The model under review builds one solid part; all positions refer to its coordinate system, in mm. A direction names the side the tool comes from. Coordinates: 2 decimals unless noted, no trailing zeros. Order: outer loops, then holes, each group sorted by start corner. A loop starts at its lowest first (then second) coordinate and runs counter-clockwise, first axis right, second up. Notation, with made-up numbers: M 42.25,-10.5 L 55.25,-10.5 A19 ccw 55.25,11.5 Z; hole C -28,0 d3. An arc over 180 degrees is marked long. Answer in a Markdown table with one row per item.
from build123d import *

# Parameters (mm, degrees)
BOSS_EXTRUDE1_DEPTH = 20
SKETCH1_3_W         = 5.45
SKETCH1_3_H         = 16
SKETCH1_3_R         = 1
SKETCH1_3_W_2       = 4
SKETCH1_3_H_2       = 10
BOSS_EXTRUDE2_DEPTH = 2


with BuildPart() as part:
    # Sketch1 → Boss-Extrude1 (new body)
    # profile 1 of 2: a face of its own
    with BuildSketch(Plane(origin=(0, 0, 0), x_dir=(1, 0, 0), z_dir=(0, 1, 0))):
        with BuildLine():
            Line((-0.906603032, 3.2), (-0.906603032, 2.43874968))
            ThreePointArc((-0.906603032, 2.43874968), (1.204646468, 1.952562419), (2.143396968, 0))
            Line((2.143396968, 0), (6.193396968, 0))
            Line((6.193396968, 0), (6.193396968, 8))
            Line((6.193396968, 8), (6.193396968, 13.2))
            Line((6.193396968, 13.2), (-0.906603032, 13.2))
            Line((-0.906603032, 13.2), (-0.906603032, 3.2))
        make_face()
        with BuildLine():
            Line((5.393396968, 12.4), (5.393396968, 0.4))
            Line((5.393396968, 0.4), (2.919064839, 0.4))
            ThreePointArc((2.919064839, 0.4), (1.922948491, 2.386135967), (-0.106603032, 3.290516677))
            Line((-0.106603032, 3.290516677), (-0.106603032, 12.4))
            Line((-0.106603032, 12.4), (5.393396968, 12.4))
        make_face(mode=Mode.SUBTRACT)
    # profile 2 of 2: a face of its own
    with BuildSketch(Plane(origin=(0, 0, 0), x_dir=(1, 0, 0), z_dir=(0, 1, 0))):
        with BuildLine():
            Line((6.193396968, 0), (2.143396968, 0))
            ThreePointArc((2.143396968, 0), (1.204646468, -1.952562419), (-0.906603032, -2.43874968))
            Line((-0.906603032, -2.43874968), (-0.906603032, -3.2))
            Line((-0.906603032, -3.2), (-0.906603032, -13.2))
            Line((-0.906603032, -13.2), (6.193396968, -13.2))
            Line((6.193396968, -13.2), (6.193396968, -8))
            Line((6.193396968, -8), (6.193396968, 0))
        make_face()
        with BuildLine():
            Line((5.393396968, -12.4), (-0.106603032, -12.4))
            Line((-0.106603032, -12.4), (-0.106603032, -3.290516677))
            ThreePointArc((-0.106603032, -3.290516677), (1.922948491, -2.386135967), (2.919064839, -0.4))
            Line((2.919064839, -0.4), (5.393396968, -0.4))
            Line((5.393396968, -0.4), (5.393396968, -12.4))
        make_face(mode=Mode.SUBTRACT)
    extrude(amount=BOSS_EXTRUDE1_DEPTH)

    # Sketch1_3 → Boss-Extrude2 (add)
    # profile 1 of 3: a face of its own
    with BuildSketch(Plane(origin=(0, 0, 0), x_dir=(1, 0, 0), z_dir=(0, 1, 0))):
        with Locations((8.918396968, 0)):
            Rectangle(SKETCH1_3_W, SKETCH1_3_H)
        with Locations(Location((9.643396968, -5.75, 0), (0, 0, 270))):
            Circle(SKETCH1_3_R, mode=Mode.SUBTRACT)
        with Locations(Location((9.643396968, 5.75, 0), (0, 0, 270))):
            Circle(SKETCH1_3_R, mode=Mode.SUBTRACT)
    # profile 2 of 3: a face of its own
    with BuildSketch(Plane(origin=(0, 0, 0), x_dir=(1, 0, 0), z_dir=(0, 1, 0))):
        with Locations((-2.906603032, 8.2)):
            Rectangle(SKETCH1_3_W_2, SKETCH1_3_H_2)
        with Locations(Location((-2.906603032, 5.7, 0), (0, 0, 270))):
            Circle(SKETCH1_3_R, mode=Mode.SUBTRACT)
        with Locations(Location((-2.906603032, 10.7, 0), (0, 0, 270))):
            Circle(SKETCH1_3_R, mode=Mode.SUBTRACT)
    # profile 3 of 3: a face of its own
    with BuildSketch(Plane(origin=(0, 0, 0), x_dir=(1, 0, 0), z_dir=(0, 1, 0))):
        with Locations((-2.906603032, -8.2)):
            Rectangle(SKETCH1_3_W_2, SKETCH1_3_H_2)
        with Locations(Location((-2.906603032, -10.7, 0), (0, 0, 270))):
            Circle(SKETCH1_3_R, mode=Mode.SUBTRACT)
        with Locations(Location((-2.906603032, -5.7, 0), (0, 0, 270))):
            Circle(SKETCH1_3_R, mode=Mode.SUBTRACT)
    extrude(amount=BOSS_EXTRUDE2_DEPTH)


solid = part.part
(1) To check wall thickness, follow line 1 (X direction, y = 0.8, z = 5.7); line 2 (Z direction, x = 3.25, y = 6.25); line 3 (X direction, y = 3.25, z = 11). State the ranges of each line that lie inside material, in increasing order. Write a range as [from, to].
Report:
| item | result |
|---|---|
| line 1 | [-4.91, -3.91], [-1.91, -0.11], [5.39, 8.64], [10.64, 11.64] |
| line 2 | [-13.2, -12.4], [-0.4, 0.4], [12.4, 13.2] |
| line 3 | [-0.91, -0.11], [5.39, 6.19] |
(2) Take a section at A-A (z = -10.7). Write out the cut boundary in (x, y).
Report:
| item | result |
|---|---|
| outline | M -4.91,0 L -3.91,0 L -3.91,2 L -4.91,2 Z; M -1.91,0 L -0.11,0 L -0.11,20 L -0.91,20 L -0.91,2 L -1.91,2 Z; M 5.39,0 L 6.19,0 L 6.19,20 L 5.39,20 Z |
(3) Insertion check: P1, Ø12, axis at y = 13.5, z = 7, coming from the +X side; P2, Ø3, axis at x = -2.5, z = -6.5, coming from the +Y side; P3, Ø12, axis at y = 10, z = -7.5, coming from the -X side; P4, Ø3, axis at x = -2.91, z = 5.7, coming from the -Y side. Each pin has a flat end and moves straight along its axis. Give the tip position at first contact, or say it passes through.
Report:
| item | result |
|---|---|
| P1 | x = 6.19 |
| P2 | y = 2 |
| P3 | x = -0.91 |
| P4 | y = 0 |
(4) Machinability: for faces 1 (the flat face through (9, 2, 0)), 2 (the flat face through (-3, 1, 3.2)), 3 (the cylindrical face through (1.9, 9.86, 2.41)), which of the approach directions +Z, -Z, +X, -X, +Y, -Y give a long, thin tool a straight path to every point of the face, cutting with its end or side? Answer none if there is none.
Report:
| item | result |
|---|---|
| face 1 | +Z, -Z, +X, +Y |
| face 2 | -X, +Y, -Y |
| face 3 | +Y, -Y |
(5) Take a section at D-D (x = 7). Write out the cut boundary in (y, z).
Report:
| item | result |
|---|---|
| outline | M 0,-8 L 2,-8 L 2,8 L 0,8 Z |
(6) The part is to be moulded in two halves that separate along Z. For faces 4 (the flat face through (3, 20, 0)), 5 (the flat face through (9, 1, 8)), 6 (the flat face through (-0.107, 10, -8)), say which applies: +Z half, -Z half, draft (parallel to the pull), parting line (faces both ways), or undercut.
Report:
| item | result |
|---|---|
| face 4 | draft |
| face 5 | +Z half |
| face 6 | undercut |
(7) Take a section at B-B (y = 2.75). Write out the cut boundary in (x, z).
Report:
| item | result |
|---|---|
| outline | M -0.91,-13.2 L 6.19,-13.2 L 6.19,13.2 L -0.91,13.2 L -0.91,2.44 A2.5 cw long -0.91,-2.44 Z; hole M -0.11,-12.4 L 5.39,-12.4 L 5.39,-0.4 L 2.92,-0.4 A3.3 cw -0.11,-3.29 Z; hole M -0.11,3.29 A3.3 cw 2.92,0.4 L 5.39,0.4 L 5.39,12.4 L -0.11,12.4 Z |
(8) Take a section at C-C (z = 7.5). Write out the cut boundary in (x, y), then the cut area to 3 significant figures.
Report:
| item | result |
|---|---|
| outline | M -4.91,0 L -0.11,0 L -0.11,20 L -0.91,20 L -0.91,2 L -4.91,2 Z; M 5.39,0 L 11.64,0 L 11.64,2 L 6.19,2 L 6.19,20 L 5.39,20 Z |
| area | 50.9 mm^2 |
